Geometry check sheet. Reference: the model listing, model coordinates, mm. Coordinates: 2 decimals unless noted, no trailing zeros. Order: outer loops, then holes, each group sorted by start corner. A loop starts at its lowest first (then second) coordinate and runs counter-clockwise, first axis right, second up. Notation, with made-up numbers: (63, 71) - (95, 71) arc R16 cw to (95, 100) - close; hole circle Ø9 at (64, -33). An arc over 180 degrees is marked (long way). One line per item, written item: value. Start each with the question number.
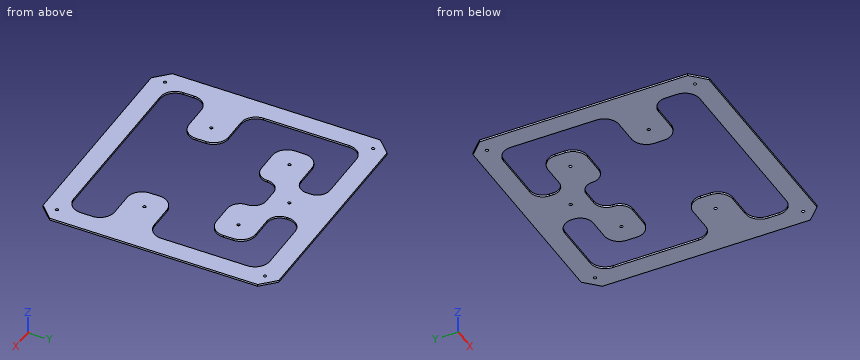
```python
from build123d import *

# Parameters (mm, degrees)
F1_DEPTH = 2
F2_D     = 3
F3_R     = 12.5
F4_DEPTH = 25


with BuildPart() as f1:
    # F0 (on Top) → F1 (new body)
    with BuildSketch(Plane.XY):
        Polygon((119, 105), (105, 119), (-105, 119), (-119, 105), (-119, -105), (-105, -119), (105, -119), (119, -105), align=None)
    extrude(amount=F1_DEPTH)

    # F2 (through all)
    with Locations(Plane(origin=(0, 0, 0), x_dir=(1, 0, 0), z_dir=(0, 0, -1))):
        with Locations((-105, -105), (105, -105), (-105, 105), (105, 105), (0, -75), (64.9519052838, 37.5), (-64.9519052838, 37.5), (-49.5, -49.5), (49.5, -49.5)):
            Hole(F2_D / 2)

    # F3 (on face) → F4 (cut)
    with BuildSketch(Plane.XY.offset(2)):
        with BuildLine():
            Line((-99, 84), (-99, -2.5))
            ThreePointArc((-99, -2.5), (-94.6066017178, -13.1066017178), (-84, -17.5))
            Line((-84, -17.5), (-59.9519052838, -17.5))
            ThreePointArc((-59.9519052838, -17.5), (-49.345303566, -21.8933982822), (-44.9519052838, -32.5))
            Line((-44.9519052838, -32.5), (-44.9519052838, -42.5))
            ThreePointArc((-44.9519052838, -42.5), (-49.345303566, -53.1066017178), (-59.9519052838, -57.5))
            Line((-59.9519052838, -57.5), (-84, -57.5))
            ThreePointArc((-84, -57.5), (-94.6066017178, -61.8933982822), (-99, -72.5))
            Line((-99, -72.5), (-99, -84))
            ThreePointArc((-99, -84), (-94.6066017178, -94.6066017178), (-84, -99))
            Line((-84, -99), (84, -99))
            ThreePointArc((84, -99), (94.6066017178, -94.6066017178), (99, -84))
            Line((99, -84), (99, -72.5))
            ThreePointArc((99, -72.5), (94.6066017178, -61.8933982822), (84, -57.5))
            Line((84, -57.5), (59.9519052838, -57.5))
            ThreePointArc((59.9519052838, -57.5), (49.345303566, -53.1066017178), (44.9519052838, -42.5))
            Line((44.9519052838, -42.5), (44.9519052838, -37.5))
            Line((44.9519052838, -37.5), (44.9519052838, -32.5))
            ThreePointArc((44.9519052838, -32.5), (49.345303566, -21.8933982822), (59.9519052838, -17.5))
            Line((59.9519052838, -17.5), (84, -17.5))
            ThreePointArc((84, -17.5), (94.6066017178, -13.1066017178), (99, -2.5))
            Line((99, -2.5), (99, 40.75))
            Line((99, 40.75), (99, 84))
            ThreePointArc((99, 84), (94.6066017178, 94.6066017178), (84, 99))
            Line((84, 99), (35, 99))
            ThreePointArc((35, 99), (24.3933982822, 94.6066017178), (20, 84))
            Line((20, 84), (20, 82.5))
            ThreePointArc((20, 82.5), (23.8076118446, 73.3076118446), (33, 69.5))
            Line((33, 69.5), (54.5, 69.5))
            ThreePointArc((54.5, 69.5), (65.1066017178, 65.1066017178), (69.5, 54.5))
            Line((69.5, 54.5), (69.5, 44.5))
            ThreePointArc((69.5, 44.5), (65.1066017178, 33.8933982822), (54.5, 29.5))
            Line((54.5, 29.5), (33, 29.5))
            ThreePointArc((33, 29.5), (23.8076118446, 33.3076118446), (20, 42.5))
            ThreePointArc((20, 42.5), (16.1923881554, 51.6923881554), (7, 55.5))
            Line((7, 55.5), (-7, 55.5))
            ThreePointArc((-7, 55.5), (-16.1923881554, 51.6923881554), (-20, 42.5))
            ThreePointArc((-20, 42.5), (-23.8076118446, 33.3076118446), (-33, 29.5))
            Line((-33, 29.5), (-54.5, 29.5))
            ThreePointArc((-54.5, 29.5), (-65.1066017178, 33.8933982822), (-69.5, 44.5))
            Line((-69.5, 44.5), (-69.5, 54.5))
            ThreePointArc((-69.5, 54.5), (-65.1066017178, 65.1066017178), (-54.5, 69.5))
            Line((-54.5, 69.5), (-33, 69.5))
            ThreePointArc((-33, 69.5), (-23.8076118446, 73.3076118446), (-20, 82.5))
            Line((-20, 82.5), (-20, 86))
            ThreePointArc((-20, 86), (-23.8076118446, 95.1923881554), (-33, 99))
            Line((-33, 99), (-84, 99))
            ThreePointArc((-84, 99), (-94.6066017178, 94.6066017178), (-99, 84))
        make_face()
        Circle(F3_R, mode=Mode.SUBTRACT)
        Circle(F3_R)
    extrude(amount=-F4_DEPTH, mode=Mode.SUBTRACT)


solid = f1.part
```
Q1. Material ranges on probe 1 along Y at (x, z) = (-85, 0.7); probe 2 along Y at (x, z) = (-105, 1.25); probe 3 along Y at (x, z) = (6, 1.6), recorded low to high.
Q2. Cross-section at B-B, the plane y = 63. Enter the section's corners in (x, z), and give its area (3 significant figures).
Q3. Cross-section at A-A, the plane y = -94. Enter the section's corners in (x, z).
Q4. Cross-section at C-C, the plane z = 1.4. Count the separate pieces of the cut face and the enclosed holes in it, and give its area (3 significant figures).
Check result:
1. probe 1: y = -119 to -98.97, -57.53 to -17.47, 98.97 to 119
1. probe 2: y = -119 to -106.5, -103.5 to 103.5, 106.5 to 119
1. probe 3: y = -119 to -99, 55.5 to 119
2. outline: (-119, 0) - (-99, 0) - (-99, 2) - (-119, 2) - close; (-66.86, 0) - (66.86, 0) - (66.86, 2) - (-66.86, 2) - close; (99, 0) - (119, 0) - (119, 2) - (99, 2) - close
2. area: 347 mm2
3. outline: (-119, 0) - (-95.18, 0) - (-95.18, 2) - (-119, 2) - close; (95.18, 0) - (119, 0) - (119, 2) - (95.18, 2) - close
4. separate pieces: 1
4. enclosed holes: 10
4. area: 27,200 mm2
